Verification items for the finished model (mm, model axes). Give positions to 0.01 mm unless a question says otherwise; leave off trailing zeros. Write each loop counter-clockwise with the first axis right and the second up, starting at its lowest first coordinate (ties: lowest second). Pieces come first, ordered by that corner, then holes. Notation, with made-up numbers: (63, 89) -> (83, 89) arc R10 ccw to (83, 94) -> close; hole circle Ø6 at (-9.5, 19). An arc over 180 degrees is marked (long way). Use one line per item in the form item = value. Start each with the question number.
(1) Section check A-A, the plane x = 262.15. Record the cut outline in (y, z), plus the area to 3 significant figures.
(2) Section check B-B, the plane z = 0.3. State how many separate pieces and enclosed holes the cut face has, plus the area to 3 significant figures.
(3) Section check C-C, the plane x = 305. Record the cut outline in (y, z).
(4) Depth check by flat-ended pin: pin 1 Ø0.5 at (y, z) = (23.5, 1) entering from -X. Enter the tip coordinate at first touch or a pass-through.
(5) Scan lines: L1, parallel to Y at x = 232.05, z = 0.65 (1 decimal); L2, parallel to Y at x = 55, z = 1.5; L3, parallel to X at y = 29, z = 0.45. Record each from-to range of solid material in increasing order.
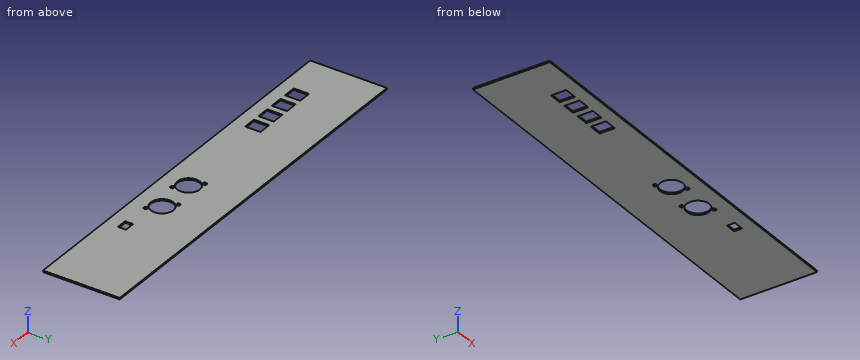
from build123d import *

# Parameters (mm, degrees)
PANEL_W             = 403
PANEL_H             = 78
BOSS_EXTRUDE1_DEPTH = 1.6
XLR4_R              = 11.5
XLR4_R_2            = 1.875
CUT_EXTRUDE2_DEPTH  = 1.6
RJ11_W              = 13.2
RJ11_H              = 15.55
CUT_EXTRUDE3_DEPTH  = 1.6
DC_PORT_W           = 10.85
DC_PORT_H           = 8.2
CUT_EXTRUDE4_DEPTH  = 1.6


with BuildPart() as part:
    # Panel → Boss-Extrude1 (new body)
    with BuildSketch(Plane.XY):
        with Locations((201.5, 39)):
            Rectangle(PANEL_W, PANEL_H)
    extrude(amount=BOSS_EXTRUDE1_DEPTH)

    # XLR4 → Cut-Extrude2 (cut)
    with BuildSketch(Plane.XY):
        with Locations(Location((222.15, 26.1, 0), (0, 0, 180))):
            Circle(XLR4_R)
        with Locations(Location((212.25, 36, 0), (0, 0, 180))):
            Circle(XLR4_R_2)
        with Locations(Location((232.05, 16.2, 0), (0, 0, 180))):
            Circle(XLR4_R_2)
        with Locations(Location((262.15, 26.1, 0), (0, 0, 180))):
            Circle(XLR4_R)
        with Locations(Location((252.25, 36, 0), (0, 0, 180))):
            Circle(XLR4_R_2)
        with Locations(Location((272.05, 16.2, 0), (0, 0, 180))):
            Circle(XLR4_R_2)
    extrude(amount=CUT_EXTRUDE2_DEPTH, mode=Mode.SUBTRACT)

    # RJ11 → Cut-Extrude3 (cut)
    with BuildSketch(Plane.XY):
        with Locations((71.2, 21.025)):
            Rectangle(RJ11_W, RJ11_H)
        with Locations((51.2, 21.025)):
            Rectangle(RJ11_W, RJ11_H)
        with Locations((91.2, 21.025)):
            Rectangle(RJ11_W, RJ11_H)
        with Locations((111.2, 21.025)):
            Rectangle(RJ11_W, RJ11_H)
    extrude(amount=CUT_EXTRUDE3_DEPTH, mode=Mode.SUBTRACT)

    # DC PORT → Cut-Extrude4 (cut)
    with BuildSketch(Plane.XY):
        with Locations((304.675, 17.65)):
            Rectangle(DC_PORT_W, DC_PORT_H)
    extrude(amount=CUT_EXTRUDE4_DEPTH, mode=Mode.SUBTRACT)


solid = part.part
Completed:
q1.outline = (0, 0) -> (14.6, 0) -> (14.6, 1.6) -> (0, 1.6) -> close; (37.6, 0) -> (78, 0) -> (78, 1.6) -> (37.6, 1.6) -> close
q1.area = 88.0 mm²
q2.separate_pieces = 1
q2.enclosed_holes = 11
q2.area = 29,600 mm²
q3.outline = (0, 0) -> (13.55, 0) -> (13.55, 1.6) -> (0, 1.6) -> close; (21.75, 0) -> (78, 0) -> (78, 1.6) -> (21.75, 1.6) -> close
q4.pin_1 = 0
q5.L1 = 0 to 14.3, 18.1 to 20.2, 32 to 78
q5.L2 = 0 to 13.25, 28.8 to 78
q5.L3 = 0 to 211.02, 233.28 to 251.02, 273.28 to 403
